Part print with two shaded views. Sizes in mm from the minimum x, y, z corner. Give positions to 0.01 mm unless a question says otherwise; leave off trailing zeros. Write each loop counter-clockwise with the first axis right and the second up, starting at its lowest first coordinate (ties: lowest second). Pieces come first, ordered by that corner, then holes. Notation, with made-up numbers: (86.25, 33.5) - (123.25, 33.5) arc R20 ccw to (123.25, 63.5) - close; hole circle Ø6 at (-19, 72.5). An arc over 180 degrees is marked (long way). One line per item, written item: value. Start each with the question number.
(1) Cut at B-B, the plane y = 26. List the corners of the cut face in (x, z).
(2) Probe L1, parallel to X at y = 4, z = 1.5; L2, parallel to X at y = 18.5, z = 5.5. List the from-to ranges inside material, lowest first.
(3) Mould opens along Y. For the marked faces 1, 2 and 3 say: pulls with the +Y half, pulls with the -Y half, needs draft (parallel to the pull), parting line crosses it, or undercut.
(4) Cut at C-C, the plane z = 21. List the corners of the cut face in (x, y).
(5) Cut at A-A, the plane x = 19. List the corners of the cut face in (y, z), and give its area (3 significant figures).
(6) Drop flat-ended pins along their axis: P1, Ø10, axis at x = 22, z = 26.5, coming from the +Y side; P2, Ø1, axis at x = 28.5, z = 17, coming from the -Y side; P3, Ø1.5, axis at x = 12.5, z = 16, coming from the +Y side. Give the stop position or say it passes through.
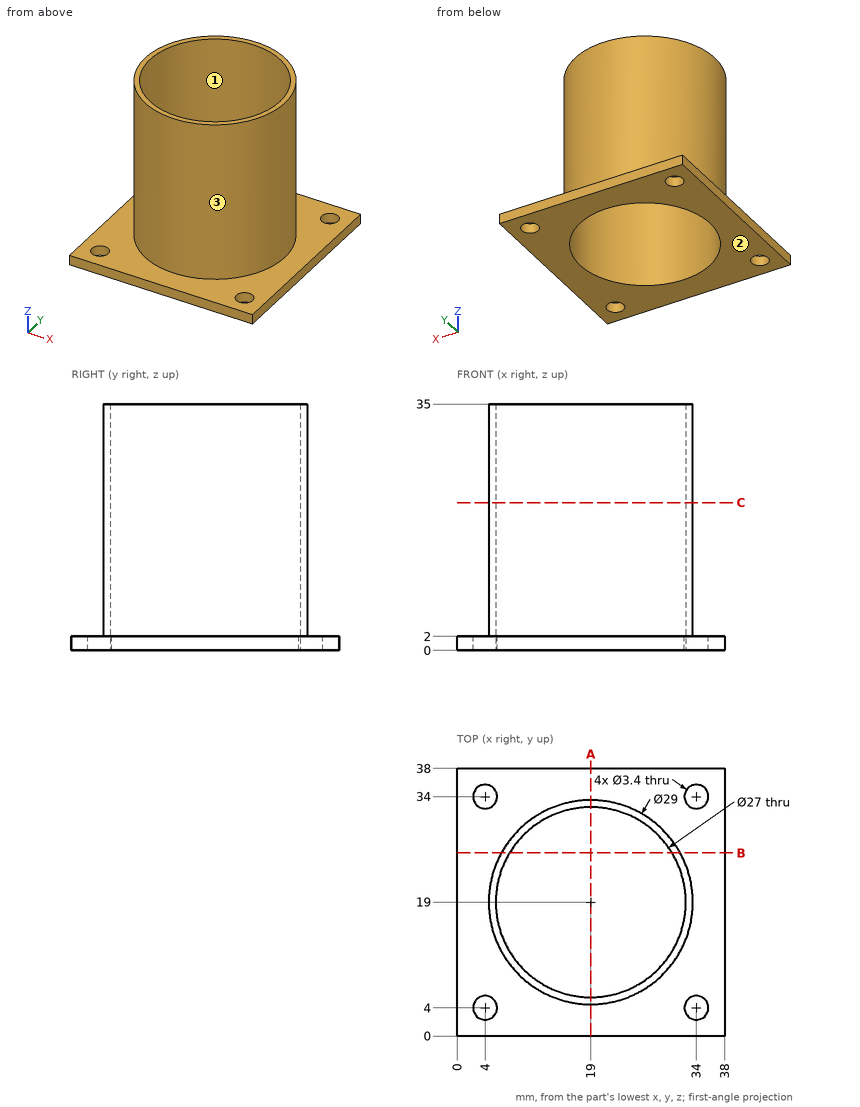
Answers follow:
1. outline: (0, 0) - (7.46, 0) - (7.46, 35) - (6.3, 35) - (6.3, 2) - (0, 2) - close; (30.54, 0) - (38, 0) - (38, 2) - (31.7, 2) - (31.7, 35) - (30.54, 35) - close
2. L1: x = 0 to 2.3, 5.7 to 32.3, 35.7 to 38
2. L2: x = 4.51 to 5.51, 32.49 to 33.49
3. face 1: undercut
3. face 2: needs draft
3. face 3: parting line crosses it
4. outline: circle Ø29 at (19, 19); hole circle Ø27 at (19, 19)
5. outline: (0, 0) - (5.5, 0) - (5.5, 35) - (4.5, 35) - (4.5, 2) - (0, 2) - close; (32.5, 0) - (38, 0) - (38, 2) - (33.5, 2) - (33.5, 35) - (32.5, 35) - close
5. area: 88.0 mm²
6. P1: stops at y = 33.5
6. P2: stops at y = 7.63
6. P3: stops at y = 32.31
